```python
from build123d import *

# Parameters (mm, degrees)
SKETCH_W      = 11
SKETCH_H      = 2.5
SKETCH_R      = 0.8
PAD_DEPTH     = 3.4
SKETCH001_W   = 13
SKETCH001_H   = 4.5
SKETCH001_W_2 = 11
SKETCH001_H_2 = 2.5
PAD001_DEPTH  = 11.9


with BuildPart() as part:
    # Sketch → Pad (new body)
    with BuildSketch(Plane.XY):
        Rectangle(SKETCH_W, SKETCH_H)
        with Locations((-1.27, 0)):
            Circle(SKETCH_R, mode=Mode.SUBTRACT)
        with Locations((1.27, 0)):
            Circle(SKETCH_R, mode=Mode.SUBTRACT)
        with Locations((3.81, 0)):
            Circle(SKETCH_R, mode=Mode.SUBTRACT)
        with Locations((-3.81, 0)):
            Circle(SKETCH_R, mode=Mode.SUBTRACT)
    extrude(amount=PAD_DEPTH)

    # Sketch001 → Pad001 (join)
    with BuildSketch(Plane.XY):
        Rectangle(SKETCH001_W, SKETCH001_H)
        Rectangle(SKETCH001_W_2, SKETCH001_H_2, mode=Mode.SUBTRACT)
    extrude(amount=PAD001_DEPTH)


solid = part.part
```
The model under review builds one solid part; all positions refer to its coordinate system, in mm. A direction names the side the tool comes from. Give positions to 0.01 mm unless a question says otherwise; leave off trailing zeros. Write each loop counter-clockwise with the first axis right and the second up, starting at its lowest first coordinate (ties: lowest second). Pieces come first, ordered by that corner, then holes. Notation, with made-up numbers: (0, 60.25) -> (10, 60.25) arc R7 cw to (10, 70.25) -> close; hole circle Ø3 at (20, -6.75). An arc over 180 degrees is marked (long way). Put each result on its own line as item: value.
(1) We need section D-D, the plane z = 2. Give the boundary of the cut face in (x, y).
Results are:
outline: (-6.5, -2.25) -> (6.5, -2.25) -> (6.5, 2.25) -> (-6.5, 2.25) -> close; hole circle Ø1.6 at (-3.81, 0); hole circle Ø1.6 at (-1.27, 0); hole circle Ø1.6 at (1.27, 0); hole circle Ø1.6 at (3.81, 0)
(2) To check wall thickness, follow probe 1 along Y at (x, z) = (-1.27, 2.55); probe 2 along Y at (x, z) = (1.75, 10.5); probe 3 along X at (y, z) = (0.55, 4.25). State the ranges of each line that lie inside material, in increasing order. Write a range as from..to.
Results are:
probe 1: -2.25..-0.8, 0.8..2.25
probe 2: -2.25..-1.25, 1.25..2.25
probe 3: -6.5..-5.5, 5.5..6.5
(3) We need section B-B, the plane y = 0. Give the boundary of the cut face in (x, z), and give its area (3 significant figures).
Results are:
outline: (-6.5, 0) -> (-4.61, 0) -> (-4.61, 3.4) -> (-5.5, 3.4) -> (-5.5, 11.9) -> (-6.5, 11.9) -> close; (-3.01, 0) -> (-2.07, 0) -> (-2.07, 3.4) -> (-3.01, 3.4) -> close; (-0.47, 0) -> (0.47, 0) -> (0.47, 3.4) -> (-0.47, 3.4) -> close; (2.07, 0) -> (3.01, 0) -> (3.01, 3.4) -> (2.07, 3.4) -> close; (4.61, 0) -> (6.5, 0) -> (6.5, 11.9) -> (5.5, 11.9) -> (5.5, 3.4) -> (4.61, 3.4) -> close
area: 39.4 mm²
(4) For pin 1 Ø1.3 at (x, y) = (1.27, 0) entering from +Z; pin 2 Ø0.8 at (x, y) = (1, 0.5) entering from +Z, all flat-tipped, find the tip position at first contact; note any pin that passes through.
Results are:
pin 1: through
pin 2: z = 3.4
(5) The part is to be moulded in two halves that separate along X. For faces 3 (the flat face through (-6.5, 0, 6)), 4 (the flat face through (0, 0, 0)), 5 (the flat face through (6.5, 0, 6)), 6 (the flat face through (5.5, 0, 8)), say which applies: pulls with the +X half, pulls with the -X half, needs draft (parallel to the pull), parting line crosses it, or undercut.
Results are:
face 3: pulls with the -X half
face 4: needs draft
face 5: pulls with the +X half
face 6: undercut
(6) We need section A-A, the plane x = 1.75. Give the boundary of the cut face in (y, z), and give its area (3 significant figures).
Results are:
outline: (-2.25, 0) -> (-0.64, 0) -> (-0.64, 3.4) -> (-1.25, 3.4) -> (-1.25, 11.9) -> (-2.25, 11.9) -> close; (0.64, 0) -> (2.25, 0) -> (2.25, 11.9) -> (1.25, 11.9) -> (1.25, 3.4) -> (0.64, 3.4) -> close
area: 27.9 mm²
(7) Tool access review of faces 1 (the flat face through (0, -1.25, 8)), 2 (the cylindrical face through (-4.61, 0.04, 1.68)): name each direction out of +Z, -Z, +X, -X, +Y, -Y from which nothing blocks a thin tool from reaching the whole face with its end or side.
Results are:
face 1: +Z
face 2: +Z, -Z
(8) We need section C-C, the plane z = 8. Give the boundary of the cut face in (x, y), and give its area (3 significant figures).
Results are:
outline: (-6.5, -2.25) -> (6.5, -2.25) -> (6.5, 2.25) -> (-6.5, 2.25) -> close; hole (-5.5, -1.25) -> (5.5, -1.25) -> (5.5, 1.25) -> (-5.5, 1.25) -> close
area: 31.0 mm²
